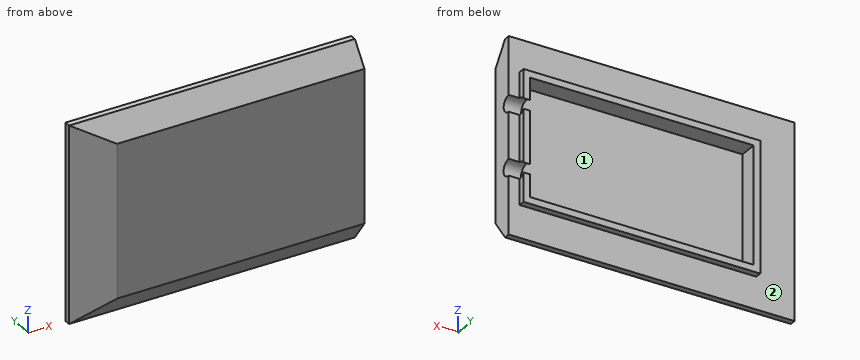
from build123d import *

# Parameters (mm, degrees)
SKETCH2_W           = 219.964
SKETCH2_H           = 149.86
SKETCH1_W           = 190.5
SKETCH1_H           = 116.84
SKETCH2_2_W         = 219.964
SKETCH2_2_H         = 149.86
BOSS_EXTRUDE2_DEPTH = 4.572
SKETCH3_W           = 182.245
SKETCH3_H           = 100.33
BOSS_EXTRUDE3_DEPTH = 5.08
SKETCH4_W           = 172.085
SKETCH4_H           = 90.17
CUT_EXTRUDE1_DEPTH  = 6.08
SKETCH4_2_W         = 172.085
SKETCH4_2_H         = 90.17
CUT_EXTRUDE2_DEPTH  = 8.89
SKETCH5_R           = 6.35
CUT_EXTRUDE3_DEPTH  = 19.05


with BuildPart() as part:
    # Sketch2 → Loft1 section 0
    with BuildSketch(Plane(origin=(0, 12.0904, 0), x_dir=(1, 0, 0), z_dir=(0, 1, 0))):
        with Locations((-109.982, -58.640869565)):
            Rectangle(SKETCH2_W, SKETCH2_H)
    # Sketch1 → Loft1 section 1
    with BuildSketch(Plane(origin=(0, 0, 0), x_dir=(1, 0, 0), z_dir=(0, 1, 0))):
        with Locations((-95.25, -58.42)):
            Rectangle(SKETCH1_W, SKETCH1_H)
    loft()

    # Sketch2_2 → Boss-Extrude2 (add)
    with BuildSketch(Plane(origin=(0, 12.0904, 0), x_dir=(1, 0, 0), z_dir=(0, 1, 0))):
        with Locations((-109.982, -58.640869565)):
            Rectangle(SKETCH2_2_W, SKETCH2_2_H)
    extrude(amount=BOSS_EXTRUDE2_DEPTH)

    # Sketch3 → Boss-Extrude3 (add)
    with BuildSketch(Plane(origin=(0, 16.51, 0), x_dir=(1, 0, 0), z_dir=(0, 1, 0))):
        with Locations((-99.5045, -58.640869565)):
            Rectangle(SKETCH3_W, SKETCH3_H)
    extrude(amount=BOSS_EXTRUDE3_DEPTH)

    # Sketch4 → Cut-Extrude1 (cut, through all)
    with BuildSketch(Plane(origin=(0, 16.51, 0), x_dir=(1, 0, 0), z_dir=(0, 1, 0))):
        with Locations((-99.5045, -58.640869565)):
            Rectangle(SKETCH4_W, SKETCH4_H)
    extrude(amount=CUT_EXTRUDE1_DEPTH, mode=Mode.SUBTRACT)

    # Sketch4_2 → Cut-Extrude2 (cut)
    with BuildSketch(Plane(origin=(0, 16.51, 0), x_dir=(1, 0, 0), z_dir=(0, 1, 0))):
        with Locations((-99.5045, -58.640869565)):
            Rectangle(SKETCH4_2_W, SKETCH4_2_H)
    extrude(amount=-CUT_EXTRUDE2_DEPTH, mode=Mode.SUBTRACT)

    # Sketch5 → Cut-Extrude3 (cut)
    with BuildSketch(Plane(origin=(0, 0, 0), x_dir=(0, 0, -1), z_dir=(1, 0, 0))):
        with Locations((-82.770869565, 16.6624)):
            Circle(SKETCH5_R)
        with Locations((-34.510869565, 16.51)):
            Circle(SKETCH5_R)
    extrude(amount=-CUT_EXTRUDE3_DEPTH, mode=Mode.SUBTRACT)


solid = part.part
Build history of the part. All positions in model axes, mm. Face numbers are marked on the shaded views. Give positions to 0.01 mm unless a question says otherwise; leave off trailing zeros. Put each result on its own line as item: value.
Item 1: Wall check: probe 1 along Z at (x, y) = (-8.75, 16.51); probe 2 along Z at (x, y) = (-28, 17.5); probe 3 along Z at (x, y) = (-78, 16). Give the ranges that are in metal, low to high.
Results are:
probe 1: -16.29 to 28.16, 40.86 to 76.42, 89.12 to 133.57
probe 2: 8.48 to 13.56, 103.73 to 108.81
probe 3: -16.29 to 13.56, 103.73 to 133.57
Item 2: Drop flat-ended pins along their axis: pin 1 Ø6 at (x, y) = (-195, 4) entering from -Z; pin 2 Ø1.5 at (x, y) = (-114, 18.5) entering from -Z; pin 3 Ø12 at (x, z) = (-92, 69) entering from +Y. Give the stop position or say it passes through.
Results are:
pin 1: z = -9.43
pin 2: z = 8.48
pin 3: y = 7.62
Item 3: Pull direction X, two halves, no side cores. Call the marked faces 1 and 2: +X half, -X half, draft (parallel to the pull), parting line (faces both ways), or undercut.
Results are:
face 1: undercut
face 2: draft
